from build123d import *

# Parameters (mm, degrees)
F0_W     = 228.6
F0_H     = 279.4
F1_DEPTH = 9.525
F3_D     = 36.5125


with BuildPart() as f1:
    # F0 (on Front) → F1 (new body, symmetric)
    with BuildSketch(Plane.XZ):
        Rectangle(F0_W, F0_H)
    extrude(amount=F1_DEPTH, both=True)

    # F3 (through all)
    with Locations(Plane.XZ.offset(9.525)):
        with Locations((0, -79.375)):
            Hole(F3_D / 2)


solid = f1.part
For this review, take the finished solid that the model builds, in its own axes (mm). Give positions to 0.01 mm unless a question says otherwise; leave off trailing zeros. Order: outer loops, then holes, each group sorted by start corner. A loop starts at its lowest first (then second) coordinate and runs counter-clockwise, first axis right, second up. Notation, with made-up numbers: (28, 84) - (59, 84) arc R14 cw to (59, 108) - close; hole circle Ø4 at (-16.5, 62.25). An arc over 180 degrees is marked (long way). Answer as a JSON object with one key per item and string values. Group by question number.
Item 1: Take a section at B-B on y = 2.5. Give the boundary of the cut face in (x, z) (1 decimal), and give its area (3 significant figures).
Item 2: Draft analysis for pull direction Z (two halves, no side actions). For faces 1 (the flat face through (-2, 0, -139.7)), 2 (the cylindrical face through (3.958, 0.133, -97.197)), 3 (the flat face through (-114.3, 0, -2)), state which applies: pulls with the +Z half, pulls with the -Z half, needs draft (parallel to the pull), parting line crosses it, or undercut.
Item 3: Wall thickness on line 1 along Z through (x, y) = (0, -2.25); line 2 along Z through (x, y) = (9.5, -7.75); line 3 along X through (y, z) = (-6, -88.5): over which ranges is each line inside the solid? List them lowest first.
Item 4: Take a section at A-A on x = 0. Give the boundary of the cut face in (y, z) (3 decimals).
Reported:
{
 "1": {"outline": "(-114.3, -139.7) - (114.3, -139.7) - (114.3, 139.7) - (-114.3, 139.7) - close; hole circle Ø36.5 at (0, -79.4)", "area": "62,800 mm^2"},
 "2": {"face 1": "pulls with the -Z half", "face 2": "undercut", "face 3": "needs draft"},
 "3": {"line 1": "-139.7 to -97.63, -61.12 to 139.7", "line 2": "-139.7 to -94.96, -63.79 to 139.7", "line 3": "-114.3 to -15.81, 15.81 to 114.3"},
 "4": {"outline": "(-9.525, -139.7) - (9.525, -139.7) - (9.525, -97.631) - (-9.525, -97.631) - close; (-9.525, -61.119) - (9.525, -61.119) - (9.525, 139.7) - (-9.525, 139.7) - close"}
}
